Read the model definition and answer for the solid it produces. Units are mm, in the model's axes. Face numbers are marked on the shaded views. A direction names the side the tool comes from. Round coordinates to 2 decimals unless told otherwise and drop trailing zeros. Write each loop counter-clockwise with the first axis right and the second up, starting at its lowest first coordinate (ties: lowest second). Pieces come first, ordered by that corner, then holes. Notation, with made-up numbers: (57.5, 54.25) -> (105.5, 54.25) arc R27 ccw to (105.5, 77.25) -> close; hole circle Ø8 at (11.25, 57.25). An arc over 180 degrees is marked (long way). Return JSON: item names as keys, results as strings.
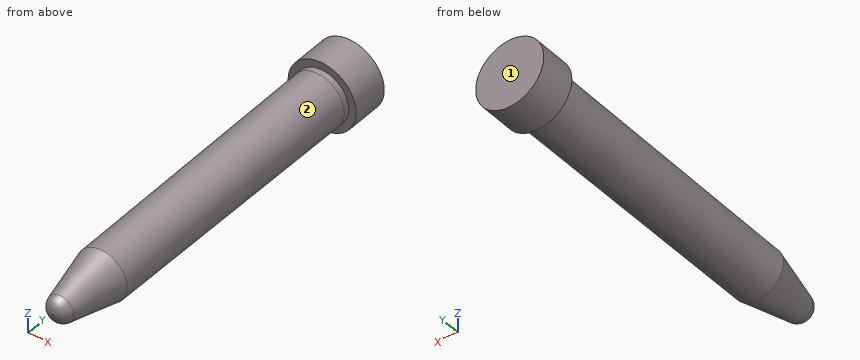
from build123d import *


# Read off the part's stored shape, not the designer's step: Shell1
with BuildPart() as part:
    # Sketch1 → Revolve1 (revolve)
    with BuildSketch(Plane.XY, mode=Mode.PRIVATE) as revolve1_sk:
        with BuildLine():
            Line((10.5, 0), (0, 0))
            Line((0, 0), (0, -117.925892815))
            Line((0, -117.925892815), (0.309007936, -117.925892815))
            ThreePointArc((0.309007936, -117.925892815), (2.721933774, -117.081420898), (4.081671516, -114.916598228))
            Line((4.081671516, -114.916598228), (7.825, -98.498944324))
            Line((7.825, -98.498944324), (8.25, -12.95))
            Line((8.25, -12.95), (8.25, -11.15))
            Line((8.25, -11.15), (10.5, -11.15))
            Line((10.5, -11.15), (10.5, 0))
        make_face()
    revolve(revolve1_sk.sketch.rotate(Axis((0, 0, 0), (0, -1, 0)), 180), axis=Axis((0, 0, 0), (0, -1, 0)))

    # Shell1 outline → Shell1 (revolve, cut)
    with BuildSketch(Plane.XY):
        with BuildLine():
            Line((0, -1), (0, -116.925892815))
            Line((0, -116.925892815), (0.309007936, -116.925892815))
            ThreePointArc((0.309007936, -116.925892815), (2.098355846, -116.299659701), (3.106693462, -114.694297092))
            Line((3.106693462, -114.694297092), (6.825559023, -98.383933749))
            Line((6.825559023, -98.383933749), (7.25, -12.947516057))
            Line((7.25, -12.947516057), (7.25, -10.15))
            Line((7.25, -10.15), (9.5, -10.15))
            Line((9.5, -10.15), (9.5, -1))
            Line((9.5, -1), (0, -1))
        make_face()
    revolve(axis=Axis((0, 0, 0), (0, 1, 0)), mode=Mode.SUBTRACT)


solid = part.part
Item 1: Straight lines are drawn through the part: L1, parallel to Z at x = 0, y = -11; L2, parallel to Z at x = 0, y = -6.5; L3, parallel to Y at x = 4.75, z = 8. For each, find the intervals that lie inside material, in ascending order. Write a range as [from, to].
Worked answers:
{"L1": "z = [-10.5, -7.25], [7.25, 10.5]", "L2": "z = [-10.5, -9.5], [9.5, 10.5]", "L3": "y = [-11.15, -10.15], [-1, 0]"}
Item 2: Section B-B (y = -74.5) is taken. Give the vertices of the cut face in (x, z), then the cut area to 3 significant figures.
Worked answers:
{"outline": "circle Ø15.89 at (0, 0); hole circle Ø13.89 at (0, 0)", "area": "46.8 mm2"}
Item 3: A tool of negligible diameter and unlimited length cuts with its end or side. For the marked faces 1 and 2, from which of +Z, -Z, +X, -X, +Y, -Y can it reach the whole face along a straight path? Write none if from no direction.
Worked answers:
{"face 1": "+Z, -Z, +X, -X, +Y", "face 2": "-Y"}
Item 4: Section A-A (y = -89) is taken. Give the vertices of the cut face in (x, z).
Worked answers:
{"outline": "circle Ø15.74 at (0, 0); hole circle Ø13.74 at (0, 0)"}
Item 5: Flat-ended cylindrical pins translate along their axes: pin 1 (4 mm diameter, centred on x = -2, z = 1.5, fed in from -Y); pin 2 (5 mm diameter, centred on y = -43, z = 1.5, fed in from +X); pin 3 (5 mm diameter, centred on y = -61, z = -1, fed in from +X). Find the tip coordinate at first contact, or state that the pin passes through.
Worked answers:
{"pin 1": "stops at y = -117.92", "pin 2": "stops at x = 8.11", "pin 3": "stops at x = 8.02"}
